```python
from build123d import *

# Parameters (mm, degrees)
SKETCH1_R           = 5.55
BASE_FLANGE1_DEPTH  = 1.5
SKETCH9_R           = 3.975
SKETCH9_R_2         = 2.475
BOSS_EXTRUDE1_DEPTH = 11.2
SKETCH11_R          = 2.475
CUT_EXTRUDE1_DEPTH  = 14.676439595


# Sheet-metal steps are written as plain solids
with BuildPart() as part:
    # Sketch1 → Base-Flange1 (new body)
    with BuildSketch(Plane.XY):
        Circle(SKETCH1_R)
    extrude(amount=-BASE_FLANGE1_DEPTH)

    # Sketch9 → Boss-Extrude1 (add)
    with BuildSketch(Plane.XY):
        Circle(SKETCH9_R)
        Circle(SKETCH9_R_2, mode=Mode.SUBTRACT)
    extrude(amount=BOSS_EXTRUDE1_DEPTH)

    # Sketch11 → Cut-Extrude1 (cut, through all)
    with BuildSketch(Plane.XY):
        Circle(SKETCH11_R)
    extrude(amount=-CUT_EXTRUDE1_DEPTH, mode=Mode.SUBTRACT)


solid = part.part
```
The listing builds one solid part. Answer for the finished solid, in the listing's coordinates (mm). A direction names the side the tool comes from. Round coordinates to 2 decimals unless told otherwise and drop trailing zeros. Order: outer loops, then holes, each group sorted by start corner. A loop starts at its lowest first (then second) coordinate and runs counter-clockwise, first axis right, second up. Notation, with made-up numbers: (16, 9) - (39, 9) arc R16 cw to (39, 27) - close; hole circle Ø11 at (28.5, 0). An arc over 180 degrees is marked (long way). Put each result on its own line as item: value. Start each with the question number.
(1) Given P1, Ø3, axis at x = -1.5, z = 5.5, coming from the -Y side (3 decimals); P2, Ø4, axis at x = 2, z = 6, coming from the +Y side (3 decimals); P3, Ø4, axis at x = 0, y = 0, coming from the +Z side; P4, Ø4, axis at x = 3.5, z = 6, coming from the +Y side, each flat-ended and moving along its own axis, determine where each tip first touches the part or whether it passes through.
(2) Find section A-A (y = 0). Give the vertices of the cut face in (x, z) (3 decimals), plus the area to 3 significant figures.
(3) For faces 1 (the flat face through (4, -2, 0)), 2 (the cylindrical face through (2.98, 4.68, -0.74)), determine the directions among +Z, -Z, +X, -X, +Y, -Y from which every point of the face is accessible in a straight line to the end or side of a thin tool.
(4) Find section C-C (z = 3.5). Give the vertices of the cut face in (x, y) (3 decimals).
(5) Straight lines are drawn through the part: probe 1 along Y at (x, z) = (0, 4) (3 decimals); probe 2 along Y at (x, z) = (0, -1.15) (3 decimals); probe 3 along X at (y, z) = (1.5, 1). For each, find the intervals that lie inside material, in ascending order. Write a range as from..to.
(6) Find section D-D (y = 2.75). Give the vertices of the cut face in (x, z).
Reply:
1. P1: y = -3.975
1. P2: y = 3.975
1. P3: through
1. P4: y = 3.68
2. outline: (-5.55, -1.5) - (-2.475, -1.5) - (-2.475, 11.2) - (-3.975, 11.2) - (-3.975, 0) - (-5.55, 0) - close; (2.475, -1.5) - (5.55, -1.5) - (5.55, 0) - (3.975, 0) - (3.975, 11.2) - (2.475, 11.2) - close
2. area: 42.8 mm^2
3. face 1: +Z
3. face 2: +Z, -Z
4. outline: circle Ø7.95 at (0, 0); hole circle Ø4.95 at (0, 0)
5. probe 1: -3.975..-2.475, 2.475..3.975
5. probe 2: -5.55..-2.475, 2.475..5.55
5. probe 3: -3.68..-1.97, 1.97..3.68
6. outline: (-4.82, -1.5) - (4.82, -1.5) - (4.82, 0) - (2.87, 0) - (2.87, 11.2) - (-2.87, 11.2) - (-2.87, 0) - (-4.82, 0) - close
